```python
from build123d import *

# Parameters (mm, degrees)
SKETCH1_R           = 7
BOSS_EXTRUDE1_DEPTH = 6.1
SKETCH2_R           = 0.75
BOSS_EXTRUDE2_DEPTH = 1
BOSS_EXTRUDE3_START = 4
SKETCH3_R           = 0.75
BOSS_EXTRUDE3_DEPTH = 4
SKETCH4_R           = 0.8
CUT_EXTRUDE1_DEPTH  = 2
SKETCH5_R           = 0.8
CUT_EXTRUDE2_DEPTH  = 2


with BuildPart() as part:
    # Sketch1 → Boss-Extrude1 (new, symmetric)
    with BuildSketch(Plane(origin=(0, 0, 0), x_dir=(1, 0, 0), z_dir=(0, 1, 0))):
        with Locations(Location((0, 0, 0), (0, 0, 270))):
            Circle(SKETCH1_R)
    extrude(amount=BOSS_EXTRUDE1_DEPTH, both=True)

    # Sketch2 → Boss-Extrude2 (add)
    with BuildSketch(Plane.XZ.offset(6.1)):
        with Locations(Location((0, 0, 0), (0, 0, 90))):
            Circle(SKETCH2_R)
    extrude(amount=BOSS_EXTRUDE2_DEPTH)

    # Sketch3 → Boss-Extrude3 (add)
    with BuildSketch(Plane(origin=(0, 6.1, 0), x_dir=(1, 0, 0), z_dir=(0, 1, 0)).offset(BOSS_EXTRUDE3_START)):
        with Locations(Location((0, 0, 0), (0, 0, 270))):
            Circle(SKETCH3_R)
    extrude(amount=-BOSS_EXTRUDE3_DEPTH)

    # Sketch4 → Cut-Extrude1 (cut)
    with BuildSketch(Plane.XZ.offset(6.1)):
        with Locations(Location((0, 4.5, 0), (0, 0, 270))):
            Circle(SKETCH4_R)
        with Locations(Location((4.5, 0, 0), (0, 0, 270))):
            Circle(SKETCH4_R)
        with Locations(Location((0, -4.5, 0), (0, 0, 270))):
            Circle(SKETCH4_R)
        with Locations(Location((-4.5, 0, 0), (0, 0, 270))):
            Circle(SKETCH4_R)
    extrude(amount=-CUT_EXTRUDE1_DEPTH, mode=Mode.SUBTRACT)

    # Sketch5 → Cut-Extrude2 (cut)
    with BuildSketch(Plane(origin=(0, 6.1, 0), x_dir=(1, 0, 0), z_dir=(0, 1, 0))):
        with Locations(Location((2.5, 0, 0), (0, 0, 270))):
            Circle(SKETCH5_R)
        with Locations(Location((0, -2.5, 0), (0, 0, 270))):
            Circle(SKETCH5_R)
        with Locations(Location((-2.5, 0, 0), (0, 0, 270))):
            Circle(SKETCH5_R)
        with Locations(Location((0, 2.5, 0), (0, 0, 270))):
            Circle(SKETCH5_R)
    extrude(amount=-CUT_EXTRUDE2_DEPTH, mode=Mode.SUBTRACT)


solid = part.part
```
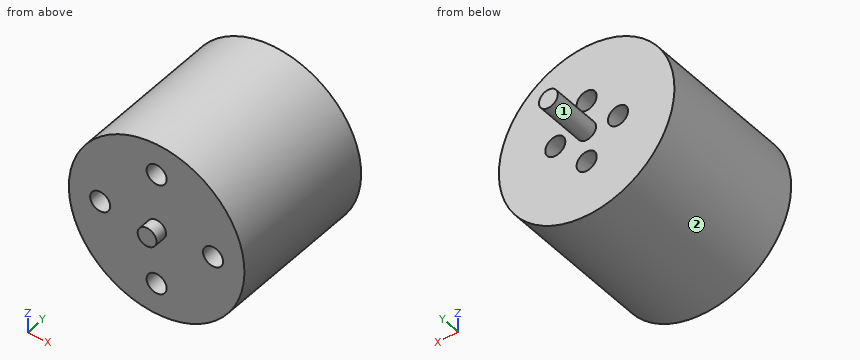
CAD build for the part. Positions are in the model's coordinates, mm. Face numbers are marked on the shaded views. A direction names the side the tool comes from. Coordinates: 2 decimals unless noted, no trailing zeros. Write each loop counter-clockwise with the first axis right and the second up, starting at its lowest first coordinate (ties: lowest second). Pieces come first, ordered by that corner, then holes. Notation, with made-up numbers: (72.5, 69) -> (86.5, 69) arc R8 ccw to (86.5, 73) -> close; hole circle Ø11 at (54.5, 68). An arc over 180 degrees is marked (long way). Use CSV: the item, a comma, the result in double quotes. Start each with the question number.
Item 1: Band-saw the part on A-A, the plane x = 0. Write the cut outline in (y, z).
Item 2: Tool access for the marked faces 1 and 2: list every direction of +Z, -Z, +X, -X, +Y, -Y with a clear straight run to the whole face (end or side of a thin tool).
Item 3: Band-saw the part on D-D, the plane z = 4.5. Write the cut outline in (x, y).
Item 4: Band-saw the part on C-C, the plane y = 7.75. Write the cut outline in (x, z).
Item 5: Band-saw the part on B-B, the plane z = 0. Write the cut outline in (x, y), plus the area to 4 significant figures.
Item 6: Wall check: probe 1 along X at (y, z) = (5, 0); probe 2 along Y at (x, z) = (2.5, -4.25); probe 3 along Y at (x, z) = (-0.5, 2). Give the ranges that are in metal, low to high.
Item 7: Drop flat-ended pins along their axis: P1, Ø1, axis at x = 2, y = 4.5, coming from the +Z side; P2, Ø0.5, axis at x = 5, z = 0, coming from the -Y side; P3, Ø1.3, axis at x = -4, z = 0, coming from the -Y side. Give the stop position or say it passes through.
Response values:
1,outline,"(-7.1, -0.75) -> (-6.1, -0.75) -> (-6.1, -3.7) -> (-4.1, -3.7) -> (-4.1, -5.3) -> (-6.1, -5.3) -> (-6.1, -7) -> (6.1, -7) -> (6.1, -3.3) -> (4.1, -3.3) -> (4.1, -1.7) -> (6.1, -1.7) -> (6.1, -0.75) -> (10.1, -0.75) -> (10.1, 0.75) -> (6.1, 0.75) -> (6.1, 1.7) -> (4.1, 1.7) -> (4.1, 3.3) -> (6.1, 3.3) -> (6.1, 7) -> (-6.1, 7) -> (-6.1, 5.3) -> (-4.1, 5.3) -> (-4.1, 3.7) -> (-6.1, 3.7) -> (-6.1, 0.75) -> (-7.1, 0.75) -> close"
2,face 1,"+Y"
2,face 2,"+Y, -Y"
3,outline,"(-5.36, -6.1) -> (-0.8, -6.1) -> (-0.8, -4.1) -> (0.8, -4.1) -> (0.8, -6.1) -> (5.36, -6.1) -> (5.36, 6.1) -> (-5.36, 6.1) -> close"
4,outline,"circle Ø1.5 at (0, 0)"
5,outline,"(-7, -6.1) -> (-5.3, -6.1) -> (-5.3, -4.1) -> (-3.7, -4.1) -> (-3.7, -6.1) -> (-0.75, -6.1) -> (-0.75, -7.1) -> (0.75, -7.1) -> (0.75, -6.1) -> (3.7, -6.1) -> (3.7, -4.1) -> (5.3, -4.1) -> (5.3, -6.1) -> (7, -6.1) -> (7, 6.1) -> (3.3, 6.1) -> (3.3, 4.1) -> (1.7, 4.1) -> (1.7, 6.1) -> (0.75, 6.1) -> (0.75, 10.1) -> (-0.75, 10.1) -> (-0.75, 6.1) -> (-1.7, 6.1) -> (-1.7, 4.1) -> (-3.3, 4.1) -> (-3.3, 6.1) -> (-7, 6.1) -> close"
5,area,"165.5 mm2"
6,probe 1,"x = -7 to -3.3, -1.7 to 1.7, 3.3 to 7"
6,probe 2,"y = -6.1 to 6.1"
6,probe 3,"y = -6.1 to 4.1"
7,P1,"stops at z = 6.84"
7,P2,"stops at y = -4.1"
7,P3,"stops at y = -6.1"
